```python
from build123d import *

# Parameters (mm, degrees)
F0_W     = 6
F0_H     = 15
F1_DEPTH = 13
F3_DEPTH = 2
F4_R     = 2.99999
F5_R     = 1
F6_R     = 1.5
F7_DEPTH = 10


# Not quite as in the source:
# - a fillet or chamfer is up to 0.001 mm smaller than in the source, because OpenCascade refuses the exact size


with BuildPart() as f1:
    # F0 (on Top) → F1 (new body)
    with BuildSketch(Plane.XY):
        with Locations((0, 7.5)):
            Rectangle(F0_W, F0_H)
    extrude(amount=F1_DEPTH)

    # F2 (on face) → F3 (join)
    with BuildSketch(Plane(origin=(0, 0, 0), x_dir=(1, 0, 0), z_dir=(0, 0, -1))):
        with BuildLine():
            ThreePointArc((-2.5, -7.5), (0, -10), (2.5, -7.5))
            Line((2.5, -7.5), (-2.5, -7.5))
        make_face()
        with BuildLine():
            Line((-2.5, -7.5), (2.5, -7.5))
            ThreePointArc((2.5, -7.5), (0, -5), (-2.5, -7.5))
        make_face()
    extrude(amount=F3_DEPTH)

    # F4 (radius 3 in the source; OpenCascade refuses exactly that, so slightly less here)
    f4_edges = [f1.edges().sort_by_distance(p)[0] for p in [
        (-3, 0, 6.5),
        (3, 0, 6.5),
        (3, 15, 6.5),
        (-3, 15, 6.5),
    ]]
    fillet(f4_edges, radius=F4_R)

    # F5
    f5_edges = [f1.edges().sort_by_distance(p)[0] for p in [
        (0, 15, 13),
        (2.121323, 14.121323, 13),
        (-2.121323, 14.121323, 13),
        (3, 7.5, 13),
        (-3, 7.5, 13),
        (2.121323, 0.878677, 13),
        (-2.121323, 0.878677, 13),
        (0, 0, 13),
    ]]
    fillet(f5_edges, radius=F5_R)

    # F6 (on Front) → F7 (cut)
    with BuildSketch(Plane.XZ):
        with Locations((0, 3.9348333655)):
            Circle(F6_R)
    extrude(amount=-F7_DEPTH, mode=Mode.SUBTRACT)


solid = f1.part
```
Can you work these out from the model? Positions are in its coordinate system, mm. A direction names the side the tool comes from. Coordinates: 2 decimals unless noted, no trailing zeros. Order: outer loops, then holes, each group sorted by start corner. A loop starts at its lowest first (then second) coordinate and runs counter-clockwise, first axis right, second up.
1. Thinking about a two-plate mould opening in Z: for faces 1 (the face through (-3, 7, 6)), 2 (the face through (0, 8, 13)), 3 (the face through (0, 10, 4)), which applies, +Z half, -Z half, draft (parallel to the pull), parting line (faces both ways), or undercut?
2. For faces 4 (the face through (-0.33, 4.93, 2.47)), 5 (the face through (-0.54, 9.94, -0.99)), 6 (the face through (2.699, 7.437, 12.715)), which set-ups out of +Z, -Z, +X, -X, +Y, -Y let a thin tool reach every point of the face, with its end or its side?
3. If we section it at B-B (y = 6.25): Please give me the cut outline in (x, z).
4. If we section it at C-C (y = 9.75): Please give me the cut outline in (x, z).
5. I need wall thicknesses on line 1 (Z direction, x = 0, y = 3.5); line 2 (X direction, y = 4.5, z = 4); line 3 (Z direction, x = 0, y = 7.5). Which ranges of each line are inside material? Lowest first, please.
6. I'm going to push flat-ended pins straight in: pin 1 (2 mm diameter, centred on y = 2.5, z = 11, fed in from +X); pin 2 (1.5 mm diameter, centred on x = -1, z = 9, fed in from -Y); pin 3 (1 mm diameter, centred on x = 2.5, z = 3.5, fed in from +Y); pin 4 (0.9 mm diameter, centred on x = 0.5, z = 3.5, fed in from -Y). Where does each tip first touch, or does it pass through?
Entries:
1. face 1: draft
1. face 2: +Z half
1. face 3: undercut
2. face 4: -Y
2. face 5: -Z
2. face 6: +Z, +X, +Y, -Y
3. outline: (-3, 0) - (-2.17, 0) - (-2.17, -2) - (2.17, -2) - (2.17, 0) - (3, 0) - (3, 12) arc R1 ccw to (2, 13) - (-2, 13) arc R1 ccw to (-3, 12) - close; hole circle Ø3 at (0, 3.93)
4. outline: (-3, 0) - (-1.09, 0) - (-1.09, -2) - (1.09, -2) - (1.09, 0) - (3, 0) - (3, 12) arc R1 ccw to (2, 13) - (-2, 13) arc R1 ccw to (-3, 12) - close; hole circle Ø3 at (0, 3.93)
5. line 1: z = 0 to 2.43, 5.43 to 13
5. line 2: x = -3 to -1.5, 1.5 to 3
5. line 3: z = -2 to 2.43, 5.43 to 13
6. pin 1: stops at x = 3
6. pin 2: stops at y = 0.01
6. pin 3: stops at y = 14.24
6. pin 4: stops at y = 10
